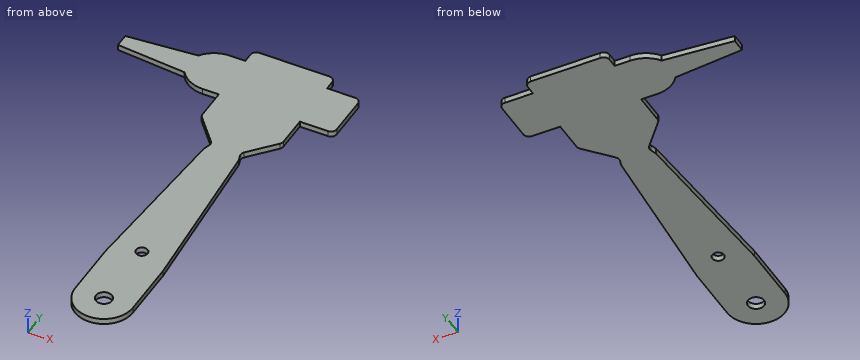
from build123d import *

# Parameters (mm, degrees)
MODEL_R           = 1
MODEL_R_2         = 1.4
BRIDA_BASE1_DEPTH = 1


# Sheet-metal steps are written as plain solids
with BuildPart() as part:
    # Model → Brida base1 (new body)
    with BuildSketch(Plane.XY):
        with BuildLine():
            Line((57.06109229, 44.40989684), (52.2059904, 44.40989684))
            Line((52.2059904, 44.40989684), (52.2059904, 46.085251303))
            ThreePointArc((52.2059904, 46.085251303), (51.913097181, 46.792358084), (51.2059904, 47.085251303))
            Line((51.2059904, 47.085251303), (39.2059904, 47.085251303))
            ThreePointArc((39.2059904, 47.085251303), (38.423096783, 46.836466455), (38.090692903, 46.085251454))
            Line((38.090692903, 46.085251454), (38.090692903, 44.40989684))
            Line((38.090692903, 44.40989684), (35.393347813, 44.40989684))
            ThreePointArc((35.393347813, 44.40989684), (32.986264566, 43.82101601), (31.122905732, 42.187392968))
            Line((31.122905732, 42.187392968), (19.054035234, 41.120549071))
            Line((19.054035234, 41.120549071), (19.054035234, 38.729385282))
            Line((19.054035234, 38.729385282), (31.122905732, 37.662541385))
            ThreePointArc((31.122905732, 37.662541385), (32.986264566, 36.028918342), (35.393347813, 35.440037512))
            Line((35.393347813, 35.440037512), (38.2059904, 35.440037512))
            Line((38.2059904, 35.440037512), (38.2059904, 30.049740987))
            ThreePointArc((38.2059904, 30.049740987), (38.270016908, 29.697670508), (38.453897645, 29.390683715))
            Line((38.453897645, 29.390683715), (42.336424948, 24.960081428))
            ThreePointArc((42.336424948, 24.960081428), (42.562673339, 24.508023196), (42.538911562, 24.0030674))
            Line((42.538911562, 24.0030674), (42.240856149, 23.048171958))
            ThreePointArc((42.240856149, 23.048171958), (42.212695742, 22.935208537), (42.197855138, 22.819737764))
            Line((42.197855138, 22.819737764), (40.2059904, -5.7615616))
            Line((40.2059904, -5.7615616), (40.2059904, -15.7615616))
            ThreePointArc((40.2059904, -15.7615616), (45.2059904, -20.7615616), (50.2059904, -15.7615616))
            Line((50.2059904, -15.7615616), (50.2059904, -5.7615616))
            Line((50.2059904, -5.7615616), (48.214125662, 22.819737764))
            ThreePointArc((48.214125662, 22.819737764), (48.199285058, 22.935208537), (48.171124651, 23.048171958))
            Line((48.171124651, 23.048171958), (47.873069238, 24.0030674))
            ThreePointArc((47.873069238, 24.0030674), (47.849307461, 24.508023196), (48.075555852, 24.960081428))
            Line((48.075555852, 24.960081428), (51.958083155, 29.390683715))
            ThreePointArc((51.958083155, 29.390683715), (52.141963892, 29.697670508), (52.2059904, 30.049740987))
            Line((52.2059904, 30.049740987), (52.2059904, 35.440037512))
            Line((52.2059904, 35.440037512), (57.06109229, 35.440037512))
            ThreePointArc((57.06109229, 35.440037512), (57.768199071, 35.732930731), (58.06109229, 36.440037513))
            Line((58.06109229, 36.440037513), (58.06109229, 43.40989684))
            ThreePointArc((58.06109229, 43.40989684), (57.768199071, 44.117003621), (57.06109229, 44.40989684))
        make_face()
        with Locations((45.2059904, -3.2615616)):
            Circle(MODEL_R, mode=Mode.SUBTRACT)
        with Locations((45.2059904, -15.7615616)):
            Circle(MODEL_R_2, mode=Mode.SUBTRACT)
    extrude(amount=-BRIDA_BASE1_DEPTH)


solid = part.part
Model file for the job. Use its own axes, mm. Give positions to 0.01 mm unless a question says otherwise; leave off trailing zeros. Loops run counter-clockwise (first coordinate to the right, second up) from the corner with the lowest first, then second, coordinate; pieces in that order, holes last.
1) Saw through at C-C (z = -0.6). Count the separate pieces of the cut face and the enclosed holes in it, plus the area to 3 significant figures.
2) Saw through at B-B (x = 30). Write the cut outline in (y, z), plus the area to 3 significant figures.
3) Saw through at A-A (y = 31). Write the cut outline in (x, z).
4) Wall check: line 1 (X direction, y = -10, z = -0.3); line 2 (X direction, y = 23, z = -0.4); line 3 (Y direction, x = 55.5, z = -0.8). Give the ranges that are in metal, low to high.
5) Flat gauge pins, fed straight in: pin 1 Ø0.5 at (x, z) = (36.5, -0.5) entering from +Y; pin 2 Ø0.5 at (x, z) = (54, -0.5) entering from -Y; pin 3 Ø10 at (x, y) = (33, -7.5) entering from +Z; pin 4 Ø0.5 at (y, z) = (45.5, -0.5) entering from +X. Where does each tip first touch, or does it go through?
Answer block:
1. separate pieces: 1
1. enclosed holes: 2
1. area: 813 mm2
2. outline: (37.76, -1) - (42.09, -1) - (42.09, 0) - (37.76, 0) - close
2. area: 4.33 mm2
3. outline: (38.21, -1) - (52.21, -1) - (52.21, 0) - (38.21, 0) - close
4. line 1: x = 40.21 to 50.21
4. line 2: x = 42.23 to 48.18
4. line 3: y = 35.44 to 44.41
5. pin 1: stops at y = 44.41
5. pin 2: stops at y = 35.44
5. pin 3: passes through
5. pin 4: stops at x = 52.21
